from build123d import *

# Parameters (mm, degrees)
BOSS_EXTRUDE1_DEPTH      = 1.4
BOSS_EXTRUDE1_DEPTH_BACK = 1
SKETCH1_R                = 12.5
SKETCH2_R                = 11.4
SKETCH2_R_2              = 10.4
BOSS_EXTRUDE2_DEPTH      = 1
CHAMFER1_SIZE            = 1
CUT_EXTRUDE6_DEPTH       = 0.4


with BuildPart() as part:
    # Sketch1 → Boss-Extrude1 (new, two sides: drawn at the far end of the back side and taken through both)
    with BuildSketch(Plane(origin=(0, 0, 0), x_dir=(1, 0, 0), z_dir=(0, 1, 0)).offset(-BOSS_EXTRUDE1_DEPTH_BACK)):
        with Locations(Location((0, 0, 0), (0, 0, 270))):
            Circle(SKETCH1_R)
    extrude(amount=BOSS_EXTRUDE1_DEPTH + BOSS_EXTRUDE1_DEPTH_BACK)

    # Sketch2 → Boss-Extrude2 (add)
    with BuildSketch(Plane(origin=(0, 1.4, 0), x_dir=(1, 0, 0), z_dir=(0, 1, 0))):
        with Locations(Location((0, 0, 0), (0, 0, 270))):
            Circle(SKETCH2_R)
        with Locations(Location((0, 0, 0), (0, 0, 270))):
            Circle(SKETCH2_R_2, mode=Mode.SUBTRACT)
    extrude(amount=BOSS_EXTRUDE2_DEPTH)

    # Chamfer1
    chamfer1_edges = [part.edges().sort_by_distance(p)[0] for p in [
        (0, -1, -12.5),
    ]]
    chamfer(chamfer1_edges, length=CHAMFER1_SIZE - 0.0001)  # a hair under: the kernel refuses the full size

    # Sketch8 → Cut-Extrude6 (cut)
    with BuildSketch(Plane.XZ.offset(1)):
        with BuildLine():
            Line((4.07421875, 4.375), (-2.1, 4.375))
            Line((-2.1, 4.375), (-2.1, 1.05))
            Line((-2.1, 1.05), (3.584765625, 1.05))
            add(Edge.make_bspline(
                [(3.584765625, 1.05), (3.683414496, 1.046266561), (3.868584149, 1.03925868), (4.127786585, 0.989689139), (4.346999538, 0.898706669), (4.525338462, 0.771743669), (4.662303563, 0.613832259), (4.762986434, 0.433813713), (4.821847618, 0.22778939), (4.828290287, 0.083326956), (4.831640625, 0.008203125)],
                knots=[0, 0, 0, 0, 1.285293232, 2.412569968, 3.418386025, 4.354403319, 5.23810445, 6.120527863, 7.022630715, 8, 8, 8, 8], degree=3))
            add(Edge.make_bspline(
                [(4.831640625, 0.008203125), (4.828384414, -0.066966736), (4.82212275, -0.211517688), (4.761888965, -0.417277321), (4.664922704, -0.60107826), (4.529268349, -0.762310942), (4.352406057, -0.893955903), (4.132637348, -0.987206532), (3.871609167, -1.039986965), (3.684368347, -1.046523103), (3.584765625, -1.05)],
                knots=[0, 0, 0, 0, 0.971200242, 1.867609123, 2.749214551, 3.645234956, 4.57279535, 5.576919765, 6.711042891, 8, 8, 8, 8], degree=3))
            Line((3.584765625, -1.05), (-2.1, -1.05))
            Line((-2.1, -1.05), (-2.1, -4.9))
            Line((-2.1, -4.9), (4.2875, -4.9))
            add(Edge.make_bspline(
                [(4.2875, -4.9), (4.388861848, -4.903792751), (4.579411283, -4.910922716), (4.847992302, -4.960158814), (5.075597112, -5.053685525), (5.263543825, -5.181722918), (5.412072035, -5.338872712), (5.514235934, -5.525740129), (5.58059817, -5.734099342), (5.586185244, -5.882024152), (5.5890625, -5.958203125)],
                knots=[0, 0, 0, 0, 1.281412047, 2.408917619, 3.431661904, 4.368016538, 5.264760761, 6.136510243, 7.040331808, 8, 8, 8, 8], degree=3))
            add(Edge.make_bspline(
                [(5.5890625, -5.958203125), (5.58633538, -6.032618077), (5.581072924, -6.176214785), (5.513038458, -6.378588348), (5.411333521, -6.561610493), (5.26351397, -6.718079765), (5.076230138, -6.847091674), (4.84693188, -6.935464254), (4.579917838, -6.99038683), (4.388974679, -6.996664043), (4.2875, -7)],
                knots=[0, 0, 0, 0, 0.944744106, 1.823049547, 2.692159438, 3.596595969, 4.540982691, 5.5681055, 6.707595947, 8, 8, 8, 8], degree=3))
            Line((4.2875, -7), (-3.1171875, -7))
            add(Edge.make_bspline(
                [(-3.1171875, -7), (-3.250668685, -6.996115514), (-3.499062513, -6.988886912), (-3.843210801, -6.9154574), (-4.13006517, -6.794002261), (-4.361921166, -6.615323708), (-4.529538591, -6.372693255), (-4.646563385, -6.075591851), (-4.711828234, -5.719439126), (-4.720407168, -5.463553728), (-4.725, -5.3265625)],
                knots=[0, 0, 0, 0, 1.189456171, 2.21344733, 3.119993849, 3.948013107, 4.78741338, 5.71757596, 6.778077714, 8, 8, 8, 8], degree=3))
            Line((-4.725, -5.3265625), (-4.725, 4.8015625))
            add(Edge.make_bspline(
                [(-4.725, 4.8015625), (-4.722897792, 4.895529375), (-4.718905933, 5.073961966), (-4.689215801, 5.328670238), (-4.638698759, 5.55670946), (-4.564380189, 5.759131594), (-4.469499051, 5.937304781), (-4.346451413, 6.088099292), (-4.199394628, 6.212046955), (-4.029553563, 6.312609172), (-3.834457239, 6.384510805), (-3.617609334, 6.440451749), (-3.374933573, 6.468369986), (-3.205653623, 6.472724382), (-3.1171875, 6.475)],
                knots=[0, 0, 0, 0, 1.257097402, 2.387087425, 3.425508426, 4.374733264, 5.264346199, 6.113849079, 6.961774747, 7.825601221, 8.740599092, 9.73444991, 10.816017894, 12, 12, 12, 12], degree=3))
            Line((-3.1171875, 6.475), (4.07421875, 6.475))
            add(Edge.make_bspline(
                [(4.07421875, 6.475), (4.176457481, 6.471126765), (4.368749199, 6.463841942), (4.638739507, 6.415846948), (4.864876279, 6.321013969), (5.050994869, 6.19434625), (5.190969541, 6.034918564), (5.297302215, 5.855179123), (5.35773805, 5.64934083), (5.364242009, 5.504673744), (5.367578125, 5.43046875)],
                knots=[0, 0, 0, 0, 1.304353081, 2.453241492, 3.474309848, 4.409392115, 5.298405909, 6.157667996, 7.055001114, 8, 8, 8, 8], degree=3))
            add(Edge.make_bspline(
                [(5.367578125, 5.43046875), (5.364372303, 5.354401915), (5.358158277, 5.206957264), (5.296483306, 4.997297579), (5.192779923, 4.813069646), (5.050706318, 4.653232754), (4.865555272, 4.525627798), (4.637979495, 4.435054103), (4.368875398, 4.385865259), (4.176501287, 4.378771597), (4.07421875, 4.375)],
                knots=[0, 0, 0, 0, 0.962139494, 1.864969442, 2.738963821, 3.622448103, 4.551714319, 5.562017248, 6.70375977, 8, 8, 8, 8], degree=3))
        make_face()
    extrude(amount=-CUT_EXTRUDE6_DEPTH, mode=Mode.SUBTRACT)


solid = part.part
Could you check a few things on this model? Use its own coordinates, in mm. A direction names the side the tool comes from. Give positions to 0.01 mm unless a question says otherwise; leave off trailing zeros. Order: outer loops, then holes, each group sorted by start corner. A loop starts at its lowest first (then second) coordinate and runs counter-clockwise, first axis right, second up. Notation, with made-up numbers: M 74,-18 L 101,-18 A6 cw 101,-9 Z; hole C 22.25,81 d4. An arc over 180 degrees is marked long. One line per question, with ' | ' between items.
1. If I drill on line 1 (X direction, y = 1.95, z = 0); line 2 (Y direction, x = 4, z = 0.5); line 3 (Y direction, x = 9, z = -4.5), over which ranges is the centre line in solid material (lowest first)?
Results:
line 1: -11.4 to -10.4, 10.4 to 11.4 | line 2: -0.6 to 1.4 | line 3: -1 to 1.4
2. I want a section at B-B (y = 2). List the corners of the cut face in (x, z) for me.
Results:
outline: C 0,0 d22.8; hole C 0,0 d20.8
3. We'd pull the mould along X, two halves only. Please class faces 3 (the face through (-10.1, 2.4, 3.3)), 4 (the face through (3.12, 1.89, 9.92)), 5 (the face through (-7, 2, -9)): +X half, -X half, draft (parallel to the pull), parting line (faces both ways), or undercut.
Results:
face 3: draft | face 4: undercut | face 5: parting line
4. I want a section at A-A (x = 0). List the corners of the cut face in (y, z) for me (3 decimals), and give its area (3 significant figures).
Results:
outline: M -1,-11.5 L 0,-12.5 L 1.4,-12.5 L 1.4,-11.4 L 2.4,-11.4 L 2.4,-10.4 L 1.4,-10.4 L 1.4,10.4 L 2.4,10.4 L 2.4,11.4 L 1.4,11.4 L 1.4,12.5 L 0,12.5 L -1,11.5 L -1,6.475 L -0.6,6.475 L -0.6,4.375 L -1,4.375 L -1,1.05 L -0.6,1.05 L -0.6,-1.05 L -1,-1.05 L -1,-4.9 L -0.6,-4.9 L -0.6,-7 L -1,-7 Z | area: 58.5 mm²
5. For faces 1 (the face through (3.755, 0.69, 11.923)), 2 (the face through (0, 1.4, 0)), which set-ups out of +Z, -Z, +X, -X, +Y, -Y let a thin tool reach every point of the face, with its end or its side?
Results:
face 1: +Y, -Y | face 2: +Y
6. I'm going to push flat-ended pins straight in: pin 1 (12.5 mm diameter, centred on x = 0, z = 1, fed in from +Y); pin 2 (2 mm diameter, centred on y = 0, z = -5.5, fed in from -X); pin 3 (2 mm diameter, centred on x = -5, y = 0.5, fed in from -Z). Where does each tip first touch, or does it pass through?
Results:
pin 1: y = 1.4 | pin 2: x = -11.66 | pin 3: z = -11.84
